Input: part model. Units: mm. Frame: model coordinates. Give positions to 0.01 mm unless a question says otherwise; leave off trailing zeros. Loops run counter-clockwise (first coordinate to the right, second up) from the corner with the lowest first, then second, coordinate; pieces in that order, holes last. Notation, with made-up numbers: (-4, 57.25) -> (21, 57.25) arc R11 cw to (21, 69.25) -> close; hole circle Ø8 at (-9.5, 42). An arc over 180 degrees is marked (long way). Answer as a JSON object with one key per item and string values.
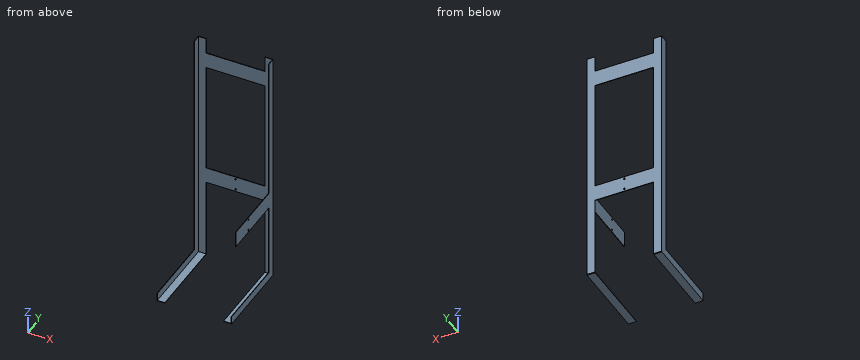
```python
from build123d import *

# Parameters (mm, degrees)
F1_DEPTH  = 1500
F3_DEPTH  = 50
F5_DEPTH  = 500
F6_W      = 3
F6_H      = 100
F9_DEPTH  = 366
F10_R     = 5
F11_DEPTH = 25
F12_W     = 3
F12_H     = 100
F13_DEPTH = 400
F14_R     = 5
F15_DEPTH = 25


with BuildPart() as f1:
    # F0 (on Top) → F1 (new body)
    with BuildSketch(Plane.XY):
        Polygon((-183, 225), (-233, 225), (-233, 175), (-230, 175), (-230, 222), (-183, 222), align=None)
    extrude(amount=F1_DEPTH)

    # F2 (on face) → F3 (join)
    with BuildSketch(Plane.YZ.offset(-183)):
        Polygon((225, 0), (222, 0), (222, -3), align=None)
    extrude(amount=-F3_DEPTH)

    # F4 (on face) → F5 (join)
    with BuildSketch(Plane.XZ.offset(-222)):
        Polygon((-233, 47), (-233, -3), (-183, -3), (-183, 0), (-230, 0), (-230, 47), align=None)
    extrude(amount=F5_DEPTH)


with BuildPart() as f8_1:
    # F8: instance of F1
    add(f1.part.mirror(Plane(origin=(0, 140.5122887865, 581.4877112135), x_dir=(0, 1, 0), z_dir=(1, 0, 0))))


with BuildPart() as f1_1:
    add(f1.part)

    add(f8_1.part)  # F9 merges F8_1
    # F6 (on face) → F9 (join, through all)
    with BuildSketch(Plane.YZ.offset(-183)):
        with Locations((223.5, 1350)):
            Rectangle(F6_W, F6_H)
        with Locations((223.5, 550)):
            Rectangle(F6_W, F6_H)
    extrude(amount=F9_DEPTH)

    # F10 (on face) → F11 (cut)
    with BuildSketch(Plane.XZ.offset(-222)):
        with Locations((0, 585)):
            Circle(F10_R)
        with Locations((0, 515)):
            Circle(F10_R)
    extrude(amount=-F11_DEPTH, mode=Mode.SUBTRACT)

    # F12 (on face) → F13 (join)
    with BuildSketch(Plane.XZ.offset(-175)):
        with Locations((231.5, 550)):
            Rectangle(F12_W, F12_H)
    extrude(amount=F13_DEPTH)

    # F14 (on face) → F15 (cut)
    with BuildSketch(Plane.YZ.offset(233)):
        with Locations((-75, 585)):
            Circle(F14_R)
        with Locations((-75, 515)):
            Circle(F14_R)
    extrude(amount=-F15_DEPTH, mode=Mode.SUBTRACT)


solid = f1_1.part
```
Q1. Ray query, line 1 along Z through (x, y) = (0, 223); line 2 along Y through (x, z) = (232.35, 515); line 3 along Y through (x, z) = (209, 1113.5). Return the intervals inside material, ascending.
Evaluation:
{"line 1": "z = 500 to 510, 520 to 580, 590 to 600, 1300 to 1400", "line 2": "y = -225 to -80, -70 to 225", "line 3": "y = 222 to 225"}
Q2. Pin query (flat end, axial travel): pin 1 (3.5 mm diameter, centred on x = -231, y = -107.5, fed in from +Z); pin 2 (5 mm diameter, centred on x = 180, z = 1005, fed in from -Y); pin 3 (2.5 mm diameter, centred on x = -232, z = 617.5, fed in from -Y); pin 4 (0.9 mm diameter, centred on x = 21.5, y = 223.5, fed in from +Z). Return the tip coordinate at first contact, or that it passes through.
Evaluation:
{"pin 1": "stops at z = 47", "pin 2": "passes through", "pin 3": "stops at y = 175", "pin 4": "stops at z = 1400"}
Q3. Section C-C, the plane y = -156.5. Return the cut outline in (x, z).
Evaluation:
{"outline": "(-233, -3) -> (-183, -3) -> (-183, 0) -> (-230, 0) -> (-230, 47) -> (-233, 47) -> close; (183, -3) -> (233, -3) -> (233, 47) -> (230, 47) -> (230, 0) -> (183, 0) -> close; (230, 500) -> (233, 500) -> (233, 600) -> (230, 600) -> close"}
Q4. Section B-B, the plane z = 757. Return the cut outline in (x, y), then the cut area to 3 significant figures.
Evaluation:
{"outline": "(-233, 175) -> (-230, 175) -> (-230, 222) -> (-183, 222) -> (-183, 225) -> (-233, 225) -> close; (183, 222) -> (230, 222) -> (230, 175) -> (233, 175) -> (233, 225) -> (183, 225) -> close", "area": "582 mm2"}
Q5. Section A-A, the plane x = 153.5. Return the cut outline in (y, z), then the cut area to 3 significant figures.
Evaluation:
{"outline": "(222, 500) -> (225, 500) -> (225, 600) -> (222, 600) -> close; (222, 1300) -> (225, 1300) -> (225, 1400) -> (222, 1400) -> close", "area": "600 mm2"}
